```python
from build123d import *

# Parameters (mm, degrees)
F1_DEPTH = 39.5986


with BuildPart() as f1:
    # F0 (on Top) → F1 (new body)
    with BuildSketch(Plane.XY):
        Polygon((36.235253, 11.773547), (37.324364, 51.372579), (0, 38.1), (-37.324364, 51.372579), (-36.235253, 11.773547), (0, 0), (22.394618, -30.823547), (60.392089, -19.622579), align=None)
        Polygon((-22.394618, -30.823547), (0, -63.5), (22.394618, -30.823547), (0, 0), (-36.235253, 11.773547), (-60.392089, -19.622579), align=None)
    extrude(amount=-F1_DEPTH)


solid = f1.part
```
Input: part model. Units: mm. Frame: model coordinates. A direction names the side the tool comes from. Coordinates: 2 decimals unless noted, no trailing zeros. Write each loop counter-clockwise with the first axis right and the second up, starting at its lowest first coordinate (ties: lowest second). Pieces come first, ordered by that corner, then holes. Notation, with made-up numbers: (72, -24) -> (106, -24) arc R23 cw to (106, 13) -> close; hole circle Ø4 at (62, -33.5). An arc over 180 degrees is marked (long way). Write each question's results on one line, items separated by ' | '.
Item 1: Mould query, pull axis X, two halves, no side actions, for faces 1 (the flat face through (18.92, 44.83, -19.52)), 2 (the flat face through (-1, -5, 0)), 3 (the flat face through (41.13, -25.3, -19.52)). Classes: +X half, -X half, draft (parallel to the pull), parting line (faces both ways), or undercut.
Conclusion:
face 1: undercut | face 2: draft | face 3: +X half
Item 2: Pin query (flat end, axial travel): pin 1 Ø3 at (x, z) = (-12.5, -23.5) entering from +Y; pin 2 Ø10 at (y, z) = (-36.5, -19) entering from -X; pin 3 Ø8 at (x, z) = (13, -35) entering from -Y. Return the tip coordinate at first contact, or that it passes through.
Conclusion:
pin 1: stops at y = 43.08 | pin 2: stops at x = -21.93 | pin 3: stops at y = -50.37
Item 3: Set-up query: faces 4 (the flat face through (11.04, -47.39, -19.52)), 5 (the flat face through (-18.401, 44.643, -19.522)). Return all of +Z, -Z, +X, -X, +Y, -Y with unobstructed straight access to the full face (end or side cutting, diameter ignored); none if empty.
Conclusion:
face 4: +Z, -Z, +X, -Y | face 5: +Z, -Z, +Y
Item 4: Section query B-B on x = 51. Return loops of the section in (y, z), plus the area to 3 significant figures.
Conclusion:
outline: (-22.39, -39.6) -> (-7.42, -39.6) -> (-7.42, 0) -> (-22.39, 0) -> close | area: 593 mm^2
Item 5: Section query C-C on y = -3.5. Return loops of the section in (x, z), plus the area to 3 significant figures.
Conclusion:
outline: (-47.99, -39.6) -> (47.99, -39.6) -> (47.99, 0) -> (-47.99, 0) -> close | area: 3,800 mm^2
Item 6: Material intervals for probe 1 along X at (y, z) = (12, -11); probe 2 along X at (y, z) = (-40.5, -1.5); probe 3 along Y at (x, z) = (7.5, -11.5), sorted ascending.
Conclusion:
probe 1: x = -36.24 to 36.24 | probe 2: x = -15.76 to 15.76 | probe 3: y = -52.56 to 40.77
Item 7: Section query A-A on z = -14. Return loops of the section in (x, y).
Conclusion:
outline: (-60.39, -19.62) -> (-22.39, -30.82) -> (0, -63.5) -> (22.39, -30.82) -> (60.39, -19.62) -> (36.24, 11.77) -> (37.32, 51.37) -> (0, 38.1) -> (-37.32, 51.37) -> (-36.24, 11.77) -> close
